The listing builds one solid part. Answer for the finished solid, in the listing's coordinates (mm). A direction names the side the tool comes from. Give positions to 0.01 mm unless a question says otherwise; leave off trailing zeros. Write each loop counter-clockwise with the first axis right and the second up, starting at its lowest first coordinate (ties: lowest second). Pieces come first, ordered by that corner, then holes. Notation, with made-up numbers: (-26.75, 85.25) -> (-12.75, 85.25) arc R31 ccw to (-12.75, 111.25) -> close; hole circle Ø4 at (29.5, 29). An arc over 180 degrees is marked (long way). Write each question's results on one line, items separated by ' | '. Start each with the question number.
from build123d import *

# Parameters (mm, degrees)
PAD_DEPTH = 5


with BuildPart() as part:
    # Sketch → Pad (new body)
    with BuildSketch(Plane.XY):
        with BuildLine():
            Line((-1.5, 22), (-1.5, -22))
            ThreePointArc((-1.5, -22), (11.5, -35), (24.5, -22))
            Line((24.5, -11), (24.5, -22))
            Line((21.5, -11), (24.5, -11))
            Line((21.5, -22), (21.5, -11))
            ThreePointArc((1.5, -22), (11.5, -32), (21.5, -22))
            Line((1.5, 22), (1.5, -22))
            ThreePointArc((1.5, 22), (-11.5, 35), (-24.5, 22))
            Line((-24.5, 11), (-24.5, 22))
            Line((-21.5, 11), (-24.5, 11))
            Line((-21.5, 22), (-21.5, 11))
            ThreePointArc((-1.5, 22), (-11.5, 32), (-21.5, 22))
        make_face()
    extrude(amount=PAD_DEPTH)


solid = part.part
1. A tool of negligible diameter and unlimited length cuts with its end or side. For faces 1 (the flat face through (-21.5, 17, 2)), 2 (the flat face through (1.5, 0, 2)), 3 (the flat face through (-23, 11, 2)), 4 (the flat face through (23, -11, 2)), from which of +Z, -Z, +X, -X, +Y, -Y can it reach the whole face along a straight path? Write none if from no direction.
2. Each of these flat-tipped pins is pushed along its axis until it touches: pin 1 Ø2 at (x, z) = (4, 2.5) entering from -Y; pin 2 Ø2.5 at (y, z) = (2.5, 3.5) entering from -X; pin 3 Ø1.5 at (y, z) = (7.5, 3.5) entering from +X. Where does it stop, or does it pass through?
3. Consider probe 1 along X at (y, z) = (19, 3.1); probe 2 along X at (y, z) = (-21.5, 0.25); probe 3 along X at (y, z) = (-8, 1.5). Determine where each line is inside the solid, lowest interval first. Write a range as [from, to].
4. Section B-B (z = 0.9) is taken. Write down the section's boundary in (x, y), then the cut area to 3 significant figures.
5. Section C-C (x = -11.5) is taken. Write down the section's boundary in (y, z), then the cut area to 3 significant figures.
6. Section A-A (y = -16.5) is taken. Write down the section's boundary in (x, z), then the cut area to 3 significant figures.
7. The mould has two halves that part along X. Classify faces 5 (the cylindrical face through (-11.3, 32, 2.5)), 6 (the flat face through (0, 0, 0)), 7 (the flat face through (24.5, -16, 2)), 8 (the cylindrical face through (11.214, -34.997, 2.465)): pulls with the +X half, pulls with the -X half, needs draft (parallel to the pull), parting line crosses it, or undercut.
8. Section D-D (y = -5.5) is taken. Write down the section's boundary in (x, z), then the cut area to 3 significant figures.
Results:
1) face 1: +Z, -Z, -Y | face 2: +Z, -Z, +Y | face 3: +Z, -Z, -X, -Y | face 4: +Z, -Z, +X, +Y
2) pin 1: stops at y = -33.26 | pin 2: stops at x = -1.5 | pin 3: stops at x = 1.5
3) probe 1: x = [-24.5, -21.5], [-1.5, 1.5] | probe 2: x = [-1.5, 1.5], [21.5, 24.5] | probe 3: x = [-1.5, 1.5]
4) outline: (-24.5, 11) -> (-21.5, 11) -> (-21.5, 22) arc R10 cw to (-1.5, 22) -> (-1.5, -22) arc R13 ccw to (24.5, -22) -> (24.5, -11) -> (21.5, -11) -> (21.5, -22) arc R10 cw to (1.5, -22) -> (1.5, 22) arc R13 ccw to (-24.5, 22) -> close | area: 415 mm²
5) outline: (32, 0) -> (35, 0) -> (35, 5) -> (32, 5) -> close | area: 15.0 mm²
6) outline: (-1.5, 0) -> (1.5, 0) -> (1.5, 5) -> (-1.5, 5) -> close; (21.5, 0) -> (24.5, 0) -> (24.5, 5) -> (21.5, 5) -> close | area: 30.0 mm²
7) face 5: undercut | face 6: needs draft | face 7: pulls with the +X half | face 8: parting line crosses it
8) outline: (-1.5, 0) -> (1.5, 0) -> (1.5, 5) -> (-1.5, 5) -> close | area: 15.0 mm²
